Autodesk Inventor part; units mm, degrees
ref_plane "YZ Plane" through (0, 0, 0) normal (1, 0, 0) x (0, 1, 0)
ref_plane "XZ Plane" through (0, 0, 0) normal (0, 1, 0) x (-1, 0, 0)
ref_plane "XY Plane" through (0, 0, 0) normal (0, 0, 1) x (1, 0, 0)
sketch "Sketch1" plane through (0, 0, 0) normal (0, 0, 1) x (1, 0, 0)
  line L0 (30, 0) -> (54, 0)
  line L1 (54, 0) -> (54, 10)
  circle A0 centre (49, 5) radius 1.6
  circle A1 centre (34, 8) radius 4
  line L2 (49, 15) -> (54, 10)
  line L3 (30, 0) -> (20, 10)
  line L4 (0, 15) -> (0, 10)
  line L5 (0, 10) -> (0, 12.5)
  line L6 (20, 10) -> (0, 10)
  line L7 (0, 15) -> (0, 17)
  line L8 (0, 17) -> (5, 17)
  line L9 (5, 17) -> (5, 15)
  line L10 (30, 15) -> (0, 15)
  line L11 (49, 15) -> (30, 15)
  line L12 (30, 15) -> (30, 15)
  point P0 (0, 0)
  dimension "d0" = 3.2
  dimension "d1" = 8
  dimension "d3" = 15
  dimension "d4" = 5
  dimension "d5" = 5
  dimension "d10" = 8
  dimension "d13" = 10
  dimension "d29" = 5
  dimension "d30" = 2
  dimension "d33" = 15
  dimension "d34" = 45
  dimension "d37" = 20
  dimension "d38" = 5
  dimension "d42" = 10
  dimension "d44" = 34
  dimension "d45" = 19
  dimension "d46" = 0
extrude "Extrusion1" add sketch "Sketch1" along normal blind 3.175
fillet "Fillet1" radius 1.5875 4 edges at (54, 10, 1.5875) (0, 10, 1.5875) (30, 0, 1.5875) (49, 15, 1.5875)
fillet "Fillet1" radius 5 1 edges at (54, 0, 1.5875)
equation "\"d7\" = THICKA"
equation "\"THICKA\" = 3.175"
equation "\"THICKB\" = 6.731"
equation "\"THICKC\" = 12.7"
equation "\"BALLDIA\" = 12"
equation "\"MAGDIA\" = 9.5"
properties part number "Air2D_Hinge_Sideplate"
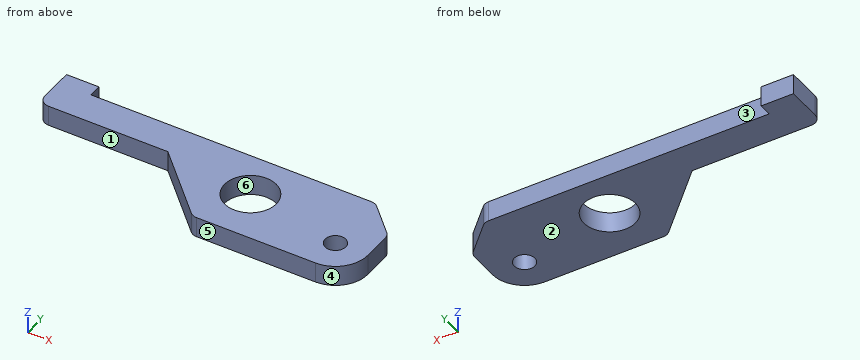
Input: part model. Units: mm. Frame: model coordinates. Face numbers are marked on the shaded views. A direction names the side the tool comes from. Coordinates: 2 decimals unless noted, no trailing zeros. Order: outer loops, then holes, each group sorted by start corner. A loop starts at its lowest first (then second) coordinate and runs counter-clockwise, first axis right, second up. Notation, with made-up numbers: (9, 66.25) - (49, 66.25) arc R31 ccw to (49, 98.25) - close; hole circle Ø1 at (-8, 57.25). An arc over 180 degrees is marked (long way). Put each result on its own line as item: value.
1. Cut plane D-D on y = 5.75. Return the cut outline in (x, z) (3 decimals).
Report:
outline: (24.25, 0) - (30.693, 0) - (30.693, 3.175) - (24.25, 3.175) - close; (37.307, 0) - (47.587, 0) - (47.587, 3.175) - (37.307, 3.175) - close; (50.413, 0) - (54, 0) - (54, 3.175) - (50.413, 3.175) - close
2. Line query: line 1 along Y through (x, z) = (34, 1.6); line 2 along X through (y, z) = (4.5, 0.8); line 3 along Y through (x, z) = (46.5, 1.4). Output: solid intervals per line, ascending.
Report:
line 1: y = 0 to 4, 12 to 15
line 2: x = 25.5 to 32.06, 35.94 to 47.48, 50.52 to 53.97
line 3: y = 0 to 15
3. Reachability of the marked faces 1, 2 and 3 from +Z, -Z, +X, -X, +Y, -Y: full face, straight path, thin tool, end or side. Return the list, or none.
Report:
face 1: +Z, -Z, -X, -Y
face 2: -Z, +X, -X, +Y, -Y
face 3: +Z, -Z, +X, +Y
4. Cut plane B-B on y = 8. Return the cut outline in (x, z) (3 decimals), then the cut area to 3 significant figures.
Report:
outline: (22, 0) - (30, 0) - (30, 3.175) - (22, 3.175) - close; (38, 0) - (54, 0) - (54, 3.175) - (38, 3.175) - close
area: 76.2 mm2
5. Contact query for flat-ended pins moving along their axis: pin 1 Ø1.6 at (y, z) = (16.5, 1.5) entering from +X; pin 2 Ø1 at (y, z) = (11.5, 1.5) entering from +X; pin 3 Ø1.5 at (x, z) = (13, 1.5) entering from +Y; pin 4 Ø8 at (x, y) = (48.5, 4) entering from +Z (3 decimals). Output: stop coordinate, or through.
Report:
pin 1: stops at x = 5
pin 2: stops at x = 53
pin 3: stops at y = 15
pin 4: stops at z = 3.175
6. Cut plane A-A on z = 1.9. Return the cut outline in (x, y) (1 decimal).
Report:
outline: (0, 11.6) arc R1.6 ccw to (1.6, 10) - (20, 10) - (29.5, 0.5) arc R1.6 ccw to (30.7, 0) - (49, 0) arc R5 ccw to (54, 5) - (54, 9.3) arc R1.6 ccw to (53.5, 10.5) - (49.5, 14.5) arc R1.6 ccw to (48.3, 15) - (5, 15) - (5, 17) - (0, 17) - close; hole circle Ø8 at (34, 8); hole circle Ø3.2 at (49, 5)
7. Draft query along X for the marked faces 4, 5 and 6. Return one class per face: pulls with the +X half, pulls with the -X half, needs draft (parallel to the pull), parting line crosses it, or undercut.
Report:
face 4: pulls with the +X half
face 5: needs draft
face 6: undercut
8. Cut plane C-C on x = 34. Return the cut outline in (y, z) (3 decimals).
Report:
outline: (0, 0) - (4, 0) - (4, 3.175) - (0, 3.175) - close; (12, 0) - (15, 0) - (15, 3.175) - (12, 3.175) - close
